The listing builds one solid part. Answer for the finished solid, in the listing's coordinates (mm). Face numbers are marked on the shaded views. A direction names the side the tool comes from. Round coordinates to 2 decimals unless told otherwise and drop trailing zeros. Order: outer loops, then holes, each group sorted by start corner. A loop starts at its lowest first (then second) coordinate and runs counter-clockwise, first axis right, second up. Notation, with made-up numbers: (68.25, -20.75) - (95.25, -20.75) arc R7 cw to (95.25, -12.75) - close; hole circle Ø2 at (76.25, 65). An arc over 180 degrees is marked (long way). Use CSV: the item, a comma, the result in double quotes. Start each with the question number.
Item 1: Find section A-A, the plane z = 13.25. Give the vertices of the cut face in (x, y), plus the area to 3 significant figures.
Item 2: Straight lines are drawn through the part: line 1 along X through (y, z) = (2.5, 13.5); line 2 along Y through (x, z) = (-10, 10); line 3 along Y through (x, z) = (-20, 13.75). For each, find the intervals that lie inside material, in ascending order. Write a range as [from, to].
Item 3: Find section B-B, the plane x = 0. Give the vertices of the cut face in (y, z).
Item 4: Find section D-D, the plane x = 20. Give the vertices of the cut face in (y, z), plus the area to 3 significant figures.
Item 5: Find section C-C, the plane y = 2.5. Give the vertices of the cut face in (x, z), plus the area to 3 significant figures.
Item 6: Flat-ended cylindrical pins translate along their axes: P1, Ø6, axis at x = -0.5, z = 12.5, coming from the -Y side; P2, Ø1.5, axis at x = 20, y = 1.5, coming from the -Z side; P3, Ø2.5, axis at y = 3.5, z = 10, coming from the +X side. Find the tip coordinate at first contact, or state that the pin passes through.
Item 7: For the marked faces 1, 2 and 3, determine the directions among +Z, -Z, +X, -X, +Y, -Y from which every point of the face is accessible in a straight line to the end or side of a thin tool.
Item 8: Determine the mould class of the marked faces 4, 5, 6 and 7 for opening direction X: +X half, -X half, draft (parallel to the pull), parting line (faces both ways), or undercut.
Autodesk Fusion 360 part; units mm, degrees
sketch "Sketch1" plane through (0, 0, 0) normal (0, 0, 1) x (1, 0, 0)
  circle A0 centre (0, 0) radius 25
  line L0 (0, 0) -> (-25, 0)
  line L1 (0, 0) -> (25, 0)
  dimension "d1" = 50
extrude "Extrude1" add sketch "Sketch1" along normal blind 20 contours A0 L0 L1 picked at (16.5736, -1.242)
sketch "Sketch2" plane through (0, 0, 0) normal (0, 1, 0) x (-1, 0, 0)
  line L0 (-25, 0) -> (25, 0)
  line L1 (25, 0) -> (25, 20)
  line L2 (25, 20) -> (-25, 20)
  line L3 (-25, 20) -> (-25, 0)
  line L4 (0, 0) -> (0, 20)
  line L5 (-25, 10) -> (25, 10)
  line L6 (0, 10) -> (-10, 10)
  line L7 (-10, 10) -> (-20, 10)
  line L8 (0, 10) -> (10, 10)
  line L9 (10, 10) -> (20, 10)
  line L10 (-17.5, 7.5) -> (-22.5, 7.5)
  line L11 (-22.5, 7.5) -> (-22.5, 12.5)
  line L12 (-22.5, 12.5) -> (-17.5, 12.5)
  line L13 (-17.5, 12.5) -> (-17.5, 7.5)
  line L14 (-17.5, 7.5) -> (-22.5, 12.5) construction
  line L15 (-22.5, 7.5) -> (-17.5, 12.5) construction
  line L16 (17.5, 12.5) -> (22.5, 12.5)
  line L17 (22.5, 12.5) -> (22.5, 7.5)
  line L18 (22.5, 7.5) -> (17.5, 7.5)
  line L19 (17.5, 7.5) -> (17.5, 12.5)
  line L20 (17.5, 12.5) -> (22.5, 7.5) construction
  line L21 (22.5, 12.5) -> (17.5, 7.5) construction
  line L22 (2.5, 7.5) -> (-2.5, 7.5)
  line L23 (-2.5, 7.5) -> (-2.5, 12.5)
  line L24 (-2.5, 12.5) -> (2.5, 12.5)
  line L25 (2.5, 12.5) -> (2.5, 7.5)
  line L26 (2.5, 7.5) -> (-2.5, 12.5) construction
  line L27 (-2.5, 7.5) -> (2.5, 12.5) construction
  point P0 (-20, 10)
  point P1 (20, 10)
  point P2 (0, 10)
  dimension "d4" = 10
  dimension "d5" = 10
  dimension "d6" = 10
  dimension "d7" = 10
  dimension "d8" = 5
  dimension "d9" = 5
  dimension "d10" = 5
  dimension "d11" = 5
  dimension "d12" = 5
  dimension "d13" = 5
extrude "Extrude2" add sketch "Sketch2" along normal blind 5 contours L4 L5 L6 L22 L23 | L4 L5 L8 L22 L25 | L5 L7 L11 L12 L13 | L5 L7 L10 L11 L13 | L4 L5 L6 L23 L24 | L4 L5 L8 L24 L25 | L5 L9 L17 L18 L19 | L5 L9 L16 L17 L19
sketch "Sketch3" plane through (0, 0, 20) normal (0, 0, 1) x (-1, 0, 0)
  arc A0 (25, 0) -> (-25, 0) centre (0, 0) ccw
  line L0 (-25, 0) -> (25, 0)
  circle A1 centre (0, 0) radius 20
  line L1 (0, 0) -> (0, 5)
  line L2 (0, 5) -> (19.3649, 5)
  line L3 (0, 5) -> (-19.3649, 5)
  dimension "d16" = 40
  dimension "d17" = 5
extrude "Extrude3" cut sketch "Sketch3" against normal blind 20 contours A1 L2 L3
sketch "Sketch4" plane through (0, 0, 12.5) normal (0, 0, 1) x (-1, 0, 0)
  line L0 (-17.5, 0) -> (-22.5, 0)
  line L1 (-22.5, 0) -> (-22.5, -5)
  line L2 (-22.5, -5) -> (-17.5, -5)
  line L3 (-17.5, -5) -> (-17.5, 0)
  circle A0 centre (-20, -2.5) radius 1
  dimension "d20" = 2
extrude "Extrude4" add sketch "Sketch4" along normal blind 3 contours A0
sketch "Sketch5" plane through (0, 0, 12.5) normal (0, 0, 1) x (-1, 0, 0)
  line L0 (2.5, 0) -> (-2.5, 0)
  line L1 (-2.5, 0) -> (-2.5, -5)
  line L2 (-2.5, -5) -> (2.5, -5)
  line L3 (2.5, -5) -> (2.5, 0)
  line L4 (0, -5) -> (0, 0)
  circle A0 centre (0, -2.5) radius 1
  dimension "d23" = 2
extrude "Extrude5" add sketch "Sketch5" along normal blind 3 contours L4 A0 | L4 A0
sketch "Sketch6" plane through (0, 0, 12.5) normal (0, 0, 1) x (-1, 0, 0)
  line L0 (22.5, 0) -> (17.5, 0)
  line L1 (17.5, 0) -> (17.5, -5)
  line L2 (17.5, -5) -> (22.5, -5)
  line L3 (22.5, -5) -> (22.5, 0)
  line L4 (20, -5) -> (20, 0)
  circle A0 centre (20, -2.5) radius 1
  dimension "d26" = 2
extrude "Extrude6" add sketch "Sketch6" along normal blind 3 contours L4 A0 | L4 A0
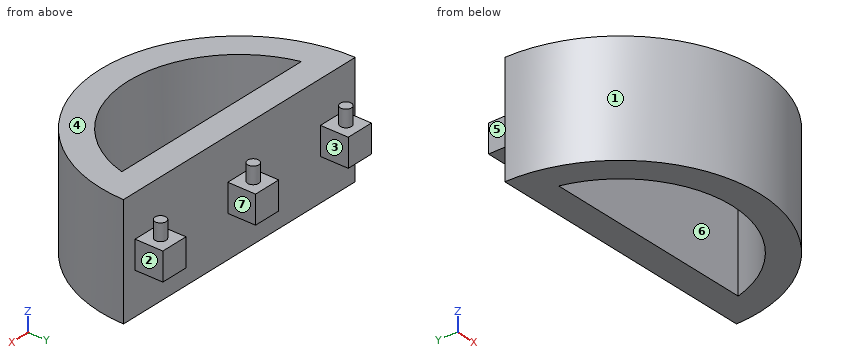
Worked out:
1,outline,"(-25, 0) arc R25 ccw to (25, 0) - close; circle Ø2 at (-20, 2.5); circle Ø2 at (0, 2.5); circle Ø2 at (20, 2.5); hole (-19.36, -5) arc R20 ccw to (19.36, -5) - close"
1,area,"561 mm²"
2,line 1,"x = [-21, -19], [-1, 1], [19, 21]"
2,line 2,"y = [-22.91, -17.32], [-5, 0]"
2,line 3,"y = [-15, 0], [1.5, 3.5]"
3,outline,"(-25, 0) - (-20, 0) - (-20, 20) - (-25, 20) - close; (-5, 0) - (0, 0) - (0, 7.5) - (5, 7.5) - (5, 12.5) - (3.5, 12.5) - (3.5, 15.5) - (1.5, 15.5) - (1.5, 12.5) - (0, 12.5) - (0, 20) - (-5, 20) - close"
4,outline,"(-15, 0) - (0, 0) - (0, 7.5) - (5, 7.5) - (5, 12.5) - (3.5, 12.5) - (3.5, 15.5) - (1.5, 15.5) - (1.5, 12.5) - (0, 12.5) - (0, 20) - (-15, 20) - close"
4,area,"331 mm²"
5,outline,"(-22.5, 7.5) - (-17.5, 7.5) - (-17.5, 12.5) - (-19, 12.5) - (-19, 15.5) - (-21, 15.5) - (-21, 12.5) - (-22.5, 12.5) - close; (-2.5, 7.5) - (2.5, 7.5) - (2.5, 12.5) - (1, 12.5) - (1, 15.5) - (-1, 15.5) - (-1, 12.5) - (-2.5, 12.5) - close; (17.5, 7.5) - (22.5, 7.5) - (22.5, 12.5) - (21, 12.5) - (21, 15.5) - (19, 15.5) - (19, 12.5) - (17.5, 12.5) - close"
5,area,"93.0 mm²"
6,P1,"stops at y = -25"
6,P2,"stops at z = 7.5"
6,P3,"stops at x = 22.5"
7,face 1,"+Z, -Z, -Y"
7,face 2,"+Z, -Z, +X, +Y"
7,face 3,"+Z, -Z, +Y"
8,face 4,"draft"
8,face 5,"-X half"
8,face 6,"undercut"
8,face 7,"undercut"
